The model under review builds one solid part; all positions refer to its coordinate system, in mm. Coordinates: 2 decimals unless noted, no trailing zeros. Write each loop counter-clockwise with the first axis right and the second up, starting at its lowest first coordinate (ties: lowest second). Pieces come first, ordered by that corner, then holes.
```python
from build123d import *

# Parameters (mm, degrees)
BASE_FLANGE1_DEPTH = 1
CUT_EXTRUDE1_DEPTH = 10
CUT_EXTRUDE2_DEPTH = 10


# Sheet-metal steps are written as plain solids
with BuildPart() as part:
    # Sketch1 → Base-Flange1 (new body)
    with BuildSketch(Plane.XY):
        with BuildLine():
            Line((0, 0), (863.4, 0))
            Line((863.4, 0), (863.4, 812))
            ThreePointArc((863.4, 812), (858.801576465, 823.101576465), (847.7, 827.7))
            Line((847.7, 827.7), (15.7, 827.7))
            ThreePointArc((15.7, 827.7), (4.598423535, 823.101576465), (0, 812))
            Line((0, 812), (0, 0))
        make_face()
    extrude(amount=-BASE_FLANGE1_DEPTH)

    # Sketch9 → Cut-Extrude1 (cut)
    with BuildSketch(Plane.XY):
        with BuildLine():
            Line((762.2, 720.7), (501.2, 720.7))
            ThreePointArc((501.2, 720.7), (499.785786438, 720.114213562), (499.2, 718.7))
            Line((499.2, 718.7), (499.2, 634.7))
            ThreePointArc((499.2, 634.7), (499.785786438, 633.285786438), (501.2, 632.7))
            Line((501.2, 632.7), (762.2, 632.7))
            ThreePointArc((762.2, 632.7), (763.614213562, 633.285786438), (764.2, 634.7))
            Line((764.2, 634.7), (764.2, 718.7))
            ThreePointArc((764.2, 718.7), (763.614213562, 720.114213562), (762.2, 720.7))
        make_face()
        with BuildLine():
            Line((764.2, 538.7), (764.2, 454.7))
            ThreePointArc((764.2, 454.7), (763.614213562, 453.285786438), (762.2, 452.7))
            Line((762.2, 452.7), (501.2, 452.7))
            ThreePointArc((501.2, 452.7), (499.785786438, 453.285786438), (499.2, 454.7))
            Line((499.2, 454.7), (499.2, 538.7))
            ThreePointArc((499.2, 538.7), (499.785786438, 540.114213562), (501.2, 540.7))
            Line((501.2, 540.7), (762.2, 540.7))
            ThreePointArc((762.2, 540.7), (763.614213562, 540.114213562), (764.2, 538.7))
        make_face()
        with BuildLine():
            Line((764.2, 358.7), (764.2, 274.7))
            ThreePointArc((764.2, 274.7), (763.614213562, 273.285786438), (762.2, 272.7))
            Line((762.2, 272.7), (501.2, 272.7))
            ThreePointArc((501.2, 272.7), (499.785786438, 273.285786438), (499.2, 274.7))
            Line((499.2, 274.7), (499.2, 358.7))
            ThreePointArc((499.2, 358.7), (499.785786438, 360.114213562), (501.2, 360.7))
            Line((501.2, 360.7), (762.2, 360.7))
            ThreePointArc((762.2, 360.7), (763.614213562, 360.114213562), (764.2, 358.7))
        make_face()
        with BuildLine():
            Line((764.2, 178.7), (764.2, 94.7))
            ThreePointArc((764.2, 94.7), (763.614213562, 93.285786438), (762.2, 92.7))
            Line((762.2, 92.7), (501.2, 92.7))
            ThreePointArc((501.2, 92.7), (499.785786438, 93.285786438), (499.2, 94.7))
            Line((499.2, 94.7), (499.2, 178.7))
            ThreePointArc((499.2, 178.7), (499.785786438, 180.114213562), (501.2, 180.7))
            Line((501.2, 180.7), (762.2, 180.7))
            ThreePointArc((762.2, 180.7), (763.614213562, 180.114213562), (764.2, 178.7))
        make_face()
        with BuildLine():
            Line((364.2, 358.7), (364.2, 274.7))
            ThreePointArc((364.2, 274.7), (363.614213562, 273.285786438), (362.2, 272.7))
            Line((362.2, 272.7), (101.2, 272.7))
            ThreePointArc((101.2, 272.7), (99.785786438, 273.285786438), (99.2, 274.7))
            Line((99.2, 274.7), (99.2, 358.7))
            ThreePointArc((99.2, 358.7), (99.785786438, 360.114213562), (101.2, 360.7))
            Line((101.2, 360.7), (362.2, 360.7))
            ThreePointArc((362.2, 360.7), (363.614213562, 360.114213562), (364.2, 358.7))
        make_face()
        with BuildLine():
            Line((364.2, 178.7), (364.2, 94.7))
            ThreePointArc((364.2, 94.7), (363.614213562, 93.285786438), (362.2, 92.7))
            Line((362.2, 92.7), (101.2, 92.7))
            ThreePointArc((101.2, 92.7), (99.785786438, 93.285786438), (99.2, 94.7))
            Line((99.2, 94.7), (99.2, 178.7))
            ThreePointArc((99.2, 178.7), (99.785786438, 180.114213562), (101.2, 180.7))
            Line((101.2, 180.7), (362.2, 180.7))
            ThreePointArc((362.2, 180.7), (363.614213562, 180.114213562), (364.2, 178.7))
        make_face()
    extrude(amount=-CUT_EXTRUDE1_DEPTH, mode=Mode.SUBTRACT)

    # Sketch10 → Cut-Extrude2 (cut)
    with BuildSketch(Plane.XY):
        with BuildLine():
            Line((91.7, 449.2), (371.7, 449.2))
            ThreePointArc((371.7, 449.2), (378.771067812, 452.128932188), (381.7, 459.2))
            Line((381.7, 459.2), (381.7, 709.2))
            ThreePointArc((381.7, 709.2), (378.771067812, 716.271067812), (371.7, 719.2))
            Line((371.7, 719.2), (91.7, 719.2))
            ThreePointArc((91.7, 719.2), (84.628932188, 716.271067812), (81.7, 709.2))
            Line((81.7, 709.2), (81.7, 459.2))
            ThreePointArc((81.7, 459.2), (84.628932188, 452.128932188), (91.7, 449.2))
        make_face()
    extrude(amount=-CUT_EXTRUDE2_DEPTH, mode=Mode.SUBTRACT)


solid = part.part
```
Item 1: Take a section at B-B, the plane y = 614.5. Write out the cut boundary in (x, z), plus the area to 3 significant figures.
Solved:
outline: (0, -1) - (81.7, -1) - (81.7, 0) - (0, 0) - close; (381.7, -1) - (863.4, -1) - (863.4, 0) - (381.7, 0) - close
area: 563 mm2
Item 2: Take a section at A-A, the plane x = 543. Write out the cut boundary in (y, z), plus the area to 3 significant figures.
Solved:
outline: (0, -1) - (92.7, -1) - (92.7, 0) - (0, 0) - close; (180.7, -1) - (272.7, -1) - (272.7, 0) - (180.7, 0) - close; (360.7, -1) - (452.7, -1) - (452.7, 0) - (360.7, 0) - close; (540.7, -1) - (632.7, -1) - (632.7, 0) - (540.7, 0) - close; (720.7, -1) - (827.7, -1) - (827.7, 0) - (720.7, 0) - close
area: 476 mm2
Item 3: Take a section at D-D, the plane y = 128.5. Write out the cut boundary in (x, z), plus the area to 3 significant figures.
Solved:
outline: (0, -1) - (99.2, -1) - (99.2, 0) - (0, 0) - close; (364.2, -1) - (499.2, -1) - (499.2, 0) - (364.2, 0) - close; (764.2, -1) - (863.4, -1) - (863.4, 0) - (764.2, 0) - close
area: 333 mm2
Item 4: To check wall thickness, follow line 1 along Y through (x, z) = (189.5, -0.7); line 2 along X through (y, z) = (503.5, -0.8); line 3 along Y through (x, z) = (547.5, -0.7). State the ranges of each line that lie inside material, in increasing order.
Solved:
line 1: y = 0 to 92.7, 180.7 to 272.7, 360.7 to 449.2, 719.2 to 827.7
line 2: x = 0 to 81.7, 381.7 to 499.2, 764.2 to 863.4
line 3: y = 0 to 92.7, 180.7 to 272.7, 360.7 to 452.7, 540.7 to 632.7, 720.7 to 827.7
Item 5: Take a section at C-C, the plane x = 252. Write out the cut boundary in (y, z).
Solved:
outline: (0, -1) - (92.7, -1) - (92.7, 0) - (0, 0) - close; (180.7, -1) - (272.7, -1) - (272.7, 0) - (180.7, 0) - close; (360.7, -1) - (449.2, -1) - (449.2, 0) - (360.7, 0) - close; (719.2, -1) - (827.7, -1) - (827.7, 0) - (719.2, 0) - close
